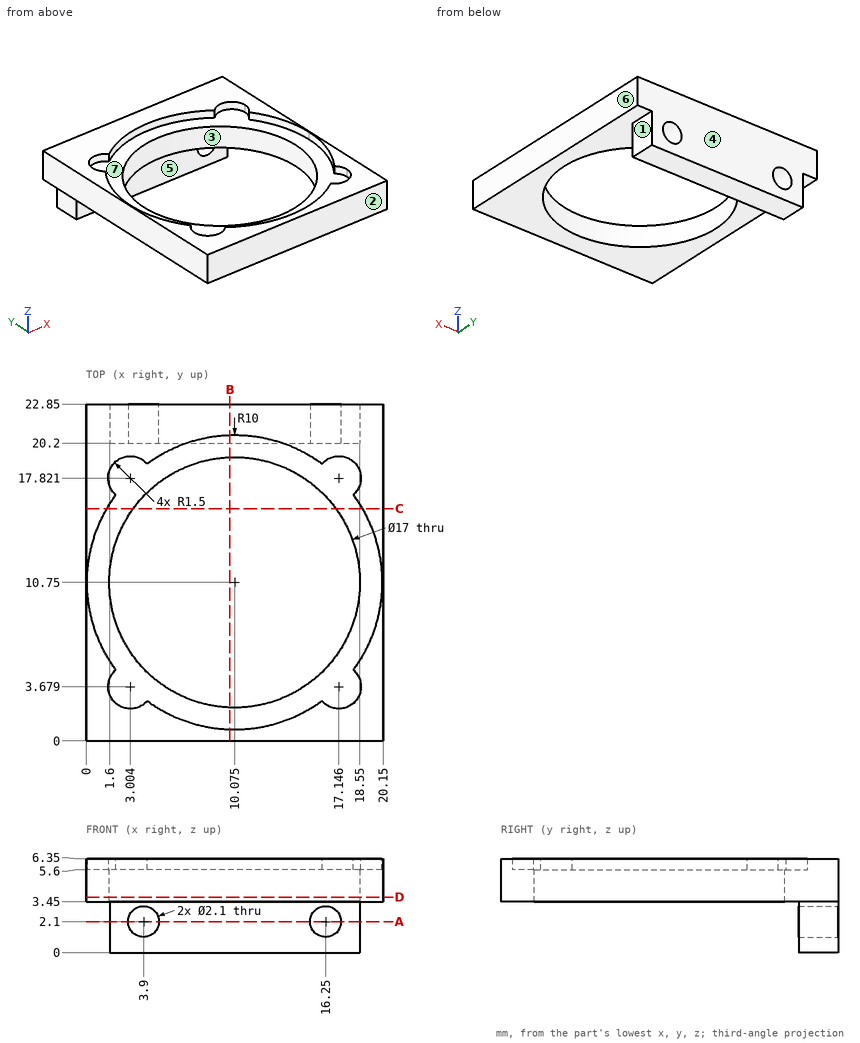
Answer from the drawing. Dimensions are ordinates in mm from the lowest x, y and z of the part. A direction names the side the tool comes from. Give positions to 0.01 mm unless a question says otherwise; leave off trailing zeros. Write each loop counter-clockwise with the first axis right and the second up, starting at its lowest first coordinate (ties: lowest second). Pieces come first, ordered by that corner, then holes.
1) Section C-C (y = 15.75) is taken. Write down the section's boundary in (x, z).
2) Section B-B (x = 9.75) is taken. Write down the section's boundary in (y, z), and give its area (3 significant figures).
3) Section D-D (z = 3.75) is taken. Write down the section's boundary in (x, y) (3 decimals).
4) Given P1, Ø2.5, axis at x = 3.9, z = 2.1, coming from the -Y side; P2, Ø5, axis at x = 2, y = 5, coming from the -Z side; P3, Ø1.9, axis at x = 16.25, z = 2.1, coming from the -Y side; P4, Ø2, axis at y = 21.5, z = 1, coming from the +X side, each flat-ended and moving along its own axis, determine where each tip first touches the part or whether it passes through.
5) Find the intervals of material crossed by L1, parallel to X at y = 10.75, z = 4.6 (3 decimals); L2, parallel to Y at x = 13.75, z = 1; L3, parallel to Z at x = 16.25, y = 22.15, in increasing order.
6) For a pull along Y with two mould halves and no side action, classify the marked faces 1, 2, 3 and 4 as pulls with the +Y half, pulls with the -Y half, needs draft (parallel to the pull), parting line crosses it, or undercut.
7) A tool of negligible diameter and unlimited length cuts with its end or side. For the marked faces 5, 6 and 7, from which of +Z, -Z, +X, -X, +Y, -Y can it reach the whole face along a straight path? Write none if from no direction.
8) Section A-A (z = 2.1) is taken. Write down the section's boundary in (x, y), and give its area (3 significant figures).
Response:
1. outline: (0, 3.45) - (3.2, 3.45) - (3.2, 5.6) - (1.41, 5.6) - (1.41, 6.35) - (0, 6.35) - close; (16.95, 3.45) - (20.15, 3.45) - (20.15, 6.35) - (18.74, 6.35) - (18.74, 5.6) - (16.95, 5.6) - close
2. outline: (0, 3.45) - (2.26, 3.45) - (2.26, 5.6) - (0.76, 5.6) - (0.76, 6.35) - (0, 6.35) - close; (19.24, 3.45) - (20.2, 3.45) - (20.2, 0) - (22.85, 0) - (22.85, 6.35) - (20.74, 6.35) - (20.74, 5.6) - (19.24, 5.6) - close
2. area: 23.9 mm2
3. outline: (0, 0) - (20.15, 0) - (20.15, 22.85) - (0, 22.85) - close; hole circle Ø17 at (10.075, 10.75)
4. P1: stops at y = 20.2
4. P2: stops at z = 3.45
4. P3: passes through
4. P4: stops at x = 18.55
5. L1: x = 0 to 1.575, 18.575 to 20.15
5. L2: y = 20.2 to 22.85
5. L3: z = 0 to 1.05, 3.15 to 6.35
6. face 1: needs draft
6. face 2: pulls with the -Y half
6. face 3: undercut
6. face 4: pulls with the +Y half
7. face 5: -Z, +X, -X, -Y
7. face 6: +Z, -Z, +X, +Y, -Y
7. face 7: +Z
8. outline: (1.6, 20.2) - (2.85, 20.2) - (2.85, 22.85) - (1.6, 22.85) - close; (4.95, 20.2) - (15.2, 20.2) - (15.2, 22.85) - (4.95, 22.85) - close; (17.3, 20.2) - (18.55, 20.2) - (18.55, 22.85) - (17.3, 22.85) - close
8. area: 33.8 mm2
